Build history of the part. All positions in model axes, mm. Face numbers are marked on the shaded views. Round coordinates to 2 decimals unless told otherwise and drop trailing zeros. Write each loop counter-clockwise with the first axis right and the second up, starting at its lowest first coordinate (ties: lowest second). Pieces come first, ordered by that corner, then holes. Notation, with made-up numbers: M 19.25,-36 L 27.25,-36 A26 cw 27.25,-17 Z; hole C 78.5,80.5 d5. An arc over 180 degrees is marked long. One line per item, written item: value. Start each with the question number.
```python
from build123d import *

# Parameters (mm, degrees)
F0_W         = 114.3
F0_H         = 82.55
F1_DEPTH     = 25.4
F2_R         = 9.525
F3_DEPTH     = 45.21898
F4_R         = 5.08
F5_T1_DEPTH  = 104.14
F5_T3_DEPTH  = 72.39
F5_S7_W      = 5.08
F5_S7_H      = 5.08
F5_T8_DEPTH  = 5.08
F5_S13_W     = 5.08
F5_S13_H     = 5.08
F5_T14_DEPTH = 5.08
F5_T20_ANGLE = 90


# Not quite as in the source:
# - a fillet or chamfer that OpenCascade refuses, or shapes differently, is made with other operations: its cross-section is extruded or revolved along the edge and cut away or added


with BuildPart() as f1:
    # F0 (on Top) → F1 (new body)
    with BuildSketch(Plane.XY):
        with Locations((-13.2126640528, 15.875)):
            Rectangle(F0_W, F0_H)
    extrude(amount=F1_DEPTH)

    # F2 (on face) → F3 (cut)
    with BuildSketch(Plane.XY.offset(25.4)):
        with Locations((-13.2126640528, 22.225)):
            Circle(F2_R)
    extrude(amount=-F3_DEPTH, mode=Mode.SUBTRACT)

    # F4
    f4_edges = [f1.edges().sort_by_distance(p)[0] for p in [
        (43.937336, 57.15, 12.7),
        (-70.362664, 57.15, 12.7),
        (43.937336, -25.4, 12.7),
        (-70.362664, -25.4, 12.7),
        (-13.212664, -25.4, 25.4),
        (-70.362664, 15.875, 25.4),
        (-70.362664, 15.875, 0),
        (43.937336, 15.875, 0),
        (-13.212664, -25.4, 0),
        (-13.212664, 57.15, 0),
        (-22.737664, 22.225, 0),
    ]]
    fillet(f4_edges, radius=F4_R)

    # F5: fillet of radius 5.08 on 2 edges, made by hand

    # F5_s2 → F5_t1 (cut)
    with BuildSketch(Plane.YZ.offset(-65.2826640528)):
        with BuildLine():
            ThreePointArc((52.07, 25.4), (55.6621024484, 23.9121024484), (57.15, 20.32))
            Line((57.15, 20.32), (57.15, 25.4))
            Line((57.15, 25.4), (52.07, 25.4))
        make_face()
    extrude(amount=F5_T1_DEPTH, mode=Mode.SUBTRACT)

    # F5_s4 → F5_t3 (cut)
    with BuildSketch(Plane.XZ.offset(-52.07)):
        with BuildLine():
            ThreePointArc((43.9373359472, 20.32), (42.4494383956, 23.9121024484), (38.8573359472, 25.4))
            Line((38.8573359472, 25.4), (43.9373359472, 25.4))
            Line((43.9373359472, 25.4), (43.9373359472, 20.32))
        make_face()
    extrude(amount=F5_T3_DEPTH, mode=Mode.SUBTRACT)


with BuildPart() as f5_tool6:
    # F5_s7 → F5_t8 (new body)
    with BuildSketch(Plane.XY.offset(20.32)):
        with Locations((-67.8226640528, 54.61)):
            Rectangle(F5_S7_W, F5_S7_H)
    extrude(amount=F5_T8_DEPTH)

    # F5_s9 → F5_t10 (revolve, cut)
    with BuildSketch(Plane(origin=(-65.2826640528, 52.07, 20.32), x_dir=(0.7071067812, -0.7071067812, 0), z_dir=(-0.7071067812, -0.7071067812, 0))):
        with BuildLine():
            ThreePointArc((0, -5.08), (5.08, 0), (0, 5.08))
            Line((0, 5.08), (0, -5.08))
        make_face()
    revolve(axis=Axis((-65.2826640528, 52.07, 20.32), (0, 0, 1)), mode=Mode.SUBTRACT)


with BuildPart() as f1_1:
    add(f1.part)

    # F5_t5: cut F5_tool6
    add(f5_tool6.part, mode=Mode.SUBTRACT)


with BuildPart() as f5_tool12:
    # F5_s13 → F5_t14 (new body)
    with BuildSketch(Plane.YZ.offset(38.8573359472)):
        with Locations((-22.86, 22.86)):
            Rectangle(F5_S13_W, F5_S13_H)
    extrude(amount=F5_T14_DEPTH)

    # F5_s15 → F5_t16 (revolve, cut)
    with BuildSketch(Plane(origin=(38.8573359472, -20.32, 20.32), x_dir=(0, 0.7071067812, -0.7071067812), z_dir=(0, -0.7071067812, -0.7071067812))):
        with BuildLine():
            ThreePointArc((0, -5.08), (5.08, 0), (0, 5.08))
            Line((0, 5.08), (0, -5.08))
        make_face()
    revolve(axis=Axis((38.8573359472, -20.32, 20.32), (1, 0, 0)), mode=Mode.SUBTRACT)


with BuildPart() as f1_2:
    add(f1_1.part)

    # F5_t11: cut F5_tool12
    add(f5_tool12.part, mode=Mode.SUBTRACT)

    # F5_s17 → F5_t18 (revolve, cut)
    with BuildSketch(Plane.XZ.offset(-22.225)):
        with BuildLine():
            ThreePointArc((1.3923359472, 25.4), (-2.1997665013, 23.9121024484), (-3.6876640528, 20.32))
            Line((-3.6876640528, 20.32), (-3.6876640528, 25.4))
            Line((-3.6876640528, 25.4), (1.3923359472, 25.4))
        make_face()
    revolve(axis=Axis((-13.2126640528, 22.225, 25.4), (0, 0, 1)), mode=Mode.SUBTRACT)

    # F5_s19 → F5_t20 (revolve, cut)
    with BuildSketch(Plane.XZ.offset(-52.07)):
        with BuildLine():
            ThreePointArc((38.8573359472, 25.4), (42.4494383956, 23.9121024484), (43.9373359472, 20.32))
            Line((43.9373359472, 20.32), (43.9373359472, 25.4))
            Line((43.9373359472, 25.4), (38.8573359472, 25.4))
        make_face()
    revolve(axis=Axis((38.8573359472, 52.07, 25.4), (0, 0, 1)), revolution_arc=F5_T20_ANGLE, mode=Mode.SUBTRACT)


solid = f1_2.part
```
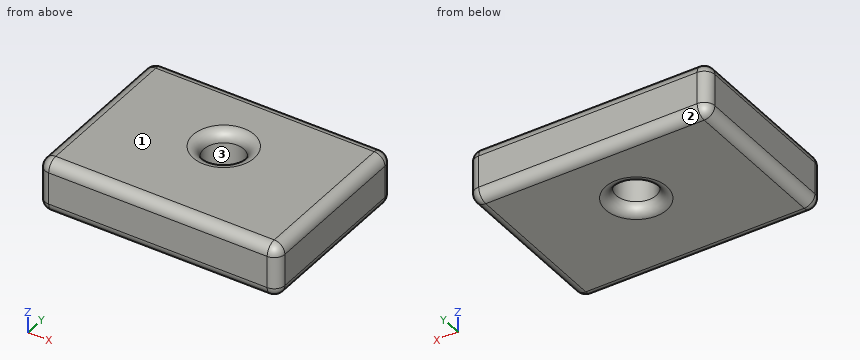
Item 1: Drop a flat-ended pin along its axis: pin 1 (1 mm diameter, centred on x = -36.5, y = 26, fed in from -Z). Give the stop position or say it passes through.
Item 2: Cut at A-A, the plane z = 17. Write the cut outline in (x, y) (3 decimals).
Item 3: Two-plate mould, pull along Y, no slides. Class the marked faces 1, 2 and 3: pulls with the +Y half, pulls with the -Y half, needs draft (parallel to the pull), parting line crosses it, or undercut.
Item 4: Drill centre lines: line 1 (Y direction, x = -6.5, z = 9.5); line 2 (X direction, y = 15.5, z = 22.25); line 3 (X direction, y = 26.5, z = 3.5). Where is each one in solid material? Low to high.
Computed values:
1. pin 1: stops at z = 0
2. outline: M -70.363,-20.32 A5.08 ccw -65.283,-25.4 L 38.857,-25.4 A5.08 ccw 43.937,-20.32 L 43.937,52.07 A5.08 ccw 38.857,57.15 L -65.283,57.15 A5.08 ccw -70.363,52.07 Z; hole C -13.213,22.225 d19.05
3. face 1: needs draft
3. face 2: pulls with the +Y half
3. face 3: undercut
4. line 1: y = -25.4 to 15.47, 28.98 to 57.15
4. line 2: x = -69.98 to -20.49, -5.94 to 43.56
4. line 3: x = -70.11 to -22.01, -4.42 to 43.69
